```python
from build123d import *

# Parameters (mm, degrees)
SKETCH1_W           = 110
SKETCH1_H           = 58
BOSS_EXTRUDE1_DEPTH = 2.5
SKETCH2_W           = 105
SKETCH2_H           = 53
BOSS_EXTRUDE2_DEPTH = 1.5
SKETCH3_W           = 7.5
SKETCH3_H           = 3
BOSS_EXTRUDE3_DEPTH = 4
FILLET1_R           = 1
SKETCH4_W           = 6
SKETCH4_H           = 2.5
CUT_EXTRUDE1_DEPTH  = 1
FILLET2_R           = 1
CHAMFER1_SIZE       = 0.5
CUT_EXTRUDE2_DEPTH  = 125.611395948
FILLET3_R           = 1
SKETCH6_R           = 1.55
CUT_EXTRUDE3_DEPTH  = 125.611395948
SKETCH7_R           = 2.05
CUT_EXTRUDE4_DEPTH  = 2


with BuildPart() as part:
    # Sketch1 → Boss-Extrude1 (new body)
    with BuildSketch(Plane(origin=(0, 0, 0), x_dir=(1, 0, 0), z_dir=(0, 1, 0))):
        with Locations((55, 29)):
            Rectangle(SKETCH1_W, SKETCH1_H)
    extrude(amount=BOSS_EXTRUDE1_DEPTH)

    # Sketch2 → Boss-Extrude2 (add)
    with BuildSketch(Plane.XZ):
        with Locations((55, -29)):
            Rectangle(SKETCH2_W, SKETCH2_H)
    extrude(amount=BOSS_EXTRUDE2_DEPTH)

    # Sketch3 → Boss-Extrude3 (add)
    with BuildSketch(Plane.XZ.offset(1.5)):
        with Locations((55, -4)):
            Rectangle(SKETCH3_W, SKETCH3_H)
        Polygon((2.5, -2.5), (10, -2.5), (10, -5.5), (5.5, -5.5), (5.5, -10), (2.5, -10), align=None)
        Polygon((107.5, -2.5), (107.5, -10), (104.5, -10), (104.5, -5.5), (100, -5.5), (100, -2.5), align=None)
        Polygon((107.5, -55.5), (100, -55.5), (100, -52.5), (104.5, -52.5), (104.5, -48), (107.5, -48), align=None)
        with Locations((55, -54)):
            Rectangle(SKETCH3_W, SKETCH3_H)
        Polygon((2.5, -55.5), (2.5, -48), (5.5, -48), (5.5, -52.5), (10, -52.5), (10, -55.5), align=None)
    extrude(amount=BOSS_EXTRUDE3_DEPTH)

    # Fillet1
    fillet1_edges = [part.edges().sort_by_distance(p)[0] for p in [
        (104.5, -3.5, -52.5),
        (5.5, -3.5, -5.5),
        (104.5, -3.5, -5.5),
        (5.5, -3.5, -52.5),
    ]]
    fillet(fillet1_edges, radius=FILLET1_R)

    # Sketch4 → Cut-Extrude1 (cut)
    with BuildSketch(Plane.XZ):
        with Locations((27.5, -1.25)):
            Rectangle(SKETCH4_W, SKETCH4_H)
        with Locations((82.5, -1.25)):
            Rectangle(SKETCH4_W, SKETCH4_H)
        with Locations((82.5, -56.75)):
            Rectangle(SKETCH4_W, SKETCH4_H)
        with Locations((27.5, -56.75)):
            Rectangle(SKETCH4_W, SKETCH4_H)
    extrude(amount=-CUT_EXTRUDE1_DEPTH, mode=Mode.SUBTRACT)

    # Fillet2
    fillet2_edges = [part.edges().sort_by_distance(p)[0] for p in [
        (0, 1.25, -58),
        (110, 1.25, -58),
        (110, 1.25, 0),
        (0, 1.25, 0),
    ]]
    fillet(fillet2_edges, radius=FILLET2_R)

    # Chamfer1
    chamfer1_edges = [part.edges().sort_by_distance(p)[0] for p in [
        (2.5, -2.75, -2.5),
        (2.5, -2.75, -55.5),
        (107.5, -2.75, -55.5),
        (107.5, -2.75, -2.5),
        (107.5, -3.5, -48),
        (100, -3.5, -55.5),
        (107.5, -5.5, -51.75),
        (103.75, -5.5, -55.5),
        (2.5, -5.5, -6.25),
        (6.25, -5.5, -2.5),
        (55, -5.5, -2.5),
        (103.75, -5.5, -2.5),
        (107.5, -5.5, -6.25),
        (55, -5.5, -55.5),
        (6.25, -5.5, -55.5),
        (2.5, -5.5, -51.75),
    ]]
    chamfer(chamfer1_edges, length=CHAMFER1_SIZE)

    # Sketch5 → Cut-Extrude2 (cut, through all)
    with BuildSketch(Plane(origin=(0, 2.5, 0), x_dir=(1, 0, 0), z_dir=(0, 1, 0))):
        with BuildLine():
            Line((28.5, 46.5), (28.5, 11.5))
            ThreePointArc((28.5, 11.5), (27.5, 10.5), (26.5, 11.5))
            Line((26.5, 11.5), (26.5, 46.5))
            ThreePointArc((26.5, 46.5), (27.5, 47.5), (28.5, 46.5))
        make_face()
        with BuildLine():
            Line((34, 46.5), (34, 11.5))
            ThreePointArc((34, 11.5), (35, 10.5), (36, 11.5))
            Line((36, 11.5), (36, 46.5))
            ThreePointArc((36, 46.5), (35, 47.5), (34, 46.5))
        make_face()
        with BuildLine():
            Line((21, 46.5), (21, 11.5))
            ThreePointArc((21, 11.5), (20, 10.5), (19, 11.5))
            Line((19, 11.5), (19, 46.5))
            ThreePointArc((19, 46.5), (20, 47.5), (21, 46.5))
        make_face()
        with BuildLine():
            Line((89, 46.5), (89, 11.5))
            ThreePointArc((89, 11.5), (90, 10.5), (91, 11.5))
            Line((91, 11.5), (91, 46.5))
            ThreePointArc((91, 46.5), (90, 47.5), (89, 46.5))
        make_face()
        with BuildLine():
            Line((74, 46.5), (74, 11.5))
            ThreePointArc((74, 11.5), (75, 10.5), (76, 11.5))
            Line((76, 11.5), (76, 46.5))
            ThreePointArc((76, 46.5), (75, 47.5), (74, 46.5))
        make_face()
        with BuildLine():
            Line((81.5, 46.5), (81.5, 11.5))
            ThreePointArc((81.5, 11.5), (82.5, 10.5), (83.5, 11.5))
            Line((83.5, 11.5), (83.5, 46.5))
            ThreePointArc((83.5, 46.5), (82.5, 47.5), (81.5, 46.5))
        make_face()
    extrude(amount=-CUT_EXTRUDE2_DEPTH, mode=Mode.SUBTRACT)

    # Fillet3
    fillet3_edges = [part.edges().sort_by_distance(p)[0] for p in [
        (0, 2.5, -29),
        (55, 2.5, -58),
        (55, 2.5, 0),
        (110, 2.5, -29),
        (109.707106781, 2.5, -0.292893219),
        (109.707106781, 2.5, -57.707106781),
        (0.292893219, 2.5, -0.292893219),
        (0.292893219, 2.5, -57.707106781),
    ]]
    fillet(fillet3_edges, radius=FILLET3_R)

    # Sketch6 → Cut-Extrude3 (cut, through all)
    with BuildSketch(Plane(origin=(0, 2.5, 0), x_dir=(1, 0, 0), z_dir=(0, 1, 0))):
        with Locations(Location((55, 29, 0), (0, 0, 270))):
            Circle(SKETCH6_R)
    extrude(amount=-CUT_EXTRUDE3_DEPTH, mode=Mode.SUBTRACT)

    # Sketch7 → Cut-Extrude4 (cut)
    with BuildSketch(Plane.XZ.offset(1.5)):
        with Locations(Location((55, -29, 0), (0, 0, 270))):
            Circle(SKETCH7_R)
    extrude(amount=-CUT_EXTRUDE4_DEPTH, mode=Mode.SUBTRACT)


solid = part.part
```
Geometry check sheet. Reference: the model listing, model coordinates, mm. A direction names the side the tool comes from. Coordinates: 2 decimals unless noted, no trailing zeros. Order: outer loops, then holes, each group sorted by start corner. A loop starts at its lowest first (then second) coordinate and runs counter-clockwise, first axis right, second up. Notation, with made-up numbers: (33.25, 61.5) - (52.25, 61.5) arc R13 cw to (52.25, 69.5) - close; hole circle Ø10 at (75, 42). An arc over 180 degrees is marked (long way). Use one line per item in the form item = value.
1. Gauge pin test, flat ends, axial feed: pin 1 (1 mm diameter, centred on y = -3, z = -8, fed in from -X); pin 2 (10 mm diameter, centred on x = 47, z = -27.5, fed in from -Y); pin 3 (1.2 mm diameter, centred on x = 83, z = -57, fed in from -Y). Record the tip position at first contact, or that the pin passes through.
Here are the results:
pin_1 = 2.5
pin_2 = -1.5
pin_3 = 1
2. Draft check along X on faces 6 (the face through (107.5, -1, -29)), 7 (the face through (27, 1, -57)), 8 (the face through (104, -5.5, -53)), 9 (the face through (83.5, 1, -29)). Enter one of: pulls with the +X half, pulls with the -X half, needs draft (parallel to the pull), parting line crosses it, or undercut.
Here are the results:
face_6 = pulls with the +X half
face_7 = undercut
face_8 = needs draft
face_9 = undercut
3. Access from +Z, -Z, +X, -X, +Y, -Y to the whole of each face (thin tool, end or side, straight path). Record for faces 1 (the face through (100, -3, -4)), 2 (the face through (27, 1, -1)), 3 (the face through (55, -5.5, -4)), 4 (the face through (74, 1, -29)), 5 (the face through (104.5, -3, -50)).
Here are the results:
face_1 = +Z, -Z, -Y
face_2 = +Z, -Y
face_3 = +Z, -Z, +X, -X, -Y
face_4 = +Y, -Y
face_5 = -Y
4. Section check B-B (z = -22.5). State how many separate pieces and enclosed holes the cut face has, then the cut area to 3 significant figures.
Here are the results:
separate_pieces = 7
enclosed_holes = 0
area = 384 mm²
5. Section check A-A (x = 35). Record the boundary of the cut face in (y, z), then the cut area to 3 significant figures.
Here are the results:
outline = (-1.5, -55.5) - (0, -55.5) - (0, -58) - (1.5, -58) arc R1 ccw to (2.5, -57) - (2.5, -47.5) - (-1.5, -47.5) - close; (-1.5, -10.5) - (2.5, -10.5) - (2.5, -1) arc R1 ccw to (1.5, 0) - (0, 0) - (0, -2.5) - (-1.5, -2.5) - close
area = 76.1 mm²
6. Scan lines: line 1 (X direction, y = -1.75, z = -9.5); line 2 (Y direction, x = 25.5, z = -35); line 3 (Z direction, x = 29, y = -0.75). Record each from-to range of solid material in increasing order.
Here are the results:
line_1 = 2.5 to 5.5, 104.5 to 107.5
line_2 = -1.5 to 2.5
line_3 = -55.5 to -2.5
